from build123d import *

# Parameters (mm, degrees)
F0_R     = 9.934414
F1_DEPTH = 25.4
F2_R     = 10.150579
F3_DEPTH = 25.4
F4_R     = 12.7


with BuildPart() as f1:
    # F0 (on Front) → F1 (new body)
    with BuildSketch(Plane.XZ):
        with BuildLine():
            Line((34.194267, 4.82379), (-53.155541, 63.962182))
            ThreePointArc((-53.155541, 63.962182), (-79.307403, 65.366782), (-92.805733, 42.92379))
            Line((-92.805733, 42.92379), (-92.805733, -7.87621))
            Line((-92.805733, -7.87621), (34.194267, -7.87621))
            Line((34.194267, -7.87621), (34.194267, 4.82379))
        make_face()
        with Locations((-67.399152, 42.92379)):
            Circle(F0_R, mode=Mode.SUBTRACT)
    extrude(amount=F1_DEPTH)

    # F2 (on face) → F3 (join)
    with BuildSketch(Plane.XZ.offset(25.4)):
        with BuildLine():
            Line((-42.007568, 4.82379), (-42.007568, 42.269981))
            ThreePointArc((-42.007568, 42.269981), (-66.745343, 68.315374), (-92.790736, 43.577599))
            Line((-92.790736, 43.577599), (-92.797315, 43.577768))
            ThreePointArc((-92.797315, 43.577768), (-92.803628, 43.250806), (-92.805733, 42.92379))
            Line((-92.805733, 42.92379), (-92.805733, 4.82379))
            Line((-92.805733, 4.82379), (-92.805733, -7.87621))
            Line((-92.805733, -7.87621), (34.194267, -7.87621))
            Line((34.194267, -7.87621), (34.194267, 4.82379))
            Line((34.194267, 4.82379), (-42.007568, 4.82379))
        make_face()
        with Locations((-67.399152, 42.92379)):
            Circle(F2_R, mode=Mode.SUBTRACT)
    extrude(amount=F3_DEPTH)

    # F4
    f4_edges = [f1.edges().sort_by_distance(p)[0] for p in [
        (34.194267, -50.8, -1.52621),
    ]]
    fillet(f4_edges, radius=F4_R)


solid = f1.part
The model under review builds one solid part; all positions refer to its coordinate system, in mm. A direction names the side the tool comes from. Round coordinates to 2 decimals unless told otherwise and drop trailing zeros. Write each loop counter-clockwise with the first axis right and the second up, starting at its lowest first coordinate (ties: lowest second). Pieces come first, ordered by that corner, then holes. Notation, with made-up numbers: M -34.5,4 L -17.5,4 A15 cw -17.5,13 Z; hole C 76,-14 d3. An arc over 180 degrees is marked long. Use a Markdown table: item, result. Add a question column.
Q1. We need section D-D, the plane y = -20. State the section outline as (x, z) points.
Q2. We need section C-C, the plane z = 35. State the section outline as (x, y) points, plus the area to 3 significant figures.
Q3. To check wall thickness, follow line 1 (X direction, y = -29, z = 7); line 2 (Z direction, x = -18.5, y = -25.5); line 3 (X direction, y = -45, z = 48.5). State the ranges of each line that lie inside material, in increasing order.
Q4. Machinability: for faces 4 (the face through (-15, -25.4, 23)), 5 (the face through (30.375, -47.178, -1.437)), which of the approach directions +Z, -Z, +X, -X, +Y, -Y give a long, thin tool a straight path to every point of the face, cutting with its end or side? Answer none if there is none.
Q5. Insertion check: pin 1 (8 mm diameter, centred on x = -34.5, z = 26, fed in from -Y); pin 2 (4 mm diameter, centred on y = -13.5, z = 39, fed in from +X); pin 3 (12.5 mm diameter, centred on y = -41, z = 22, fed in from +X). Each pin has a flat end and moves straight along its axis. Give the tip position at first contact, or say it passes through.
Q6. The part is to be moulded in two halves that separate along X. For faces 1 (the face through (34.194, -19, -2)), 2 (the face through (-3, -38, 4.824)), 3 (the face through (-57.717, -37.922, 45.973)), say which applies: pulls with the +X half, pulls with the -X half, needs draft (parallel to the pull), parting line crosses it, or undercut.
Findings below:
| question | item | result |
|---|---|---|
| 1 | outline | M -92.81,-7.88 L 34.19,-7.88 L 34.19,4.82 L -53.16,63.96 A25.41 ccw -92.81,42.92 Z; hole C -67.4,42.92 d19.87 |
| 2 | outline | M -92.81,-50.8 L -73.74,-50.8 L -73.74,-25.4 L -73.39,-25.4 L -73.39,0 L -92.81,0 Z; M -61.41,-25.4 L -61.06,-25.4 L -61.06,-50.8 L -42.01,-50.8 L -42.01,-25.4 L -10.38,-25.4 L -10.38,0 L -61.41,0 Z |
| 2 | area | 2,760 mm² |
| 3 | line 1 | x = -92.81 to -42.01 |
| 3 | line 2 | z = -7.88 to 4.82 |
| 3 | line 3 | x = -92.18 to -75.88, -58.92 to -42.62 |
| 4 | face 4 | +Z, +X, -Y |
| 4 | face 5 | +Z, -Z, +X, -Y |
| 5 | pin 1 | stops at y = -25.4 |
| 5 | pin 2 | stops at x = -13.33 |
| 5 | pin 3 | stops at x = -42.01 |
| 6 | face 1 | pulls with the +X half |
| 6 | face 2 | needs draft |
| 6 | face 3 | undercut |
